The listing builds one solid part. Answer for the finished solid, in the listing's coordinates (mm). Face numbers are marked on the shaded views. Give positions to 0.01 mm unless a question says otherwise; leave off trailing zeros. Order: outer loops, then holes, each group sorted by start corner. A loop starts at its lowest first (then second) coordinate and runs counter-clockwise, first axis right, second up.
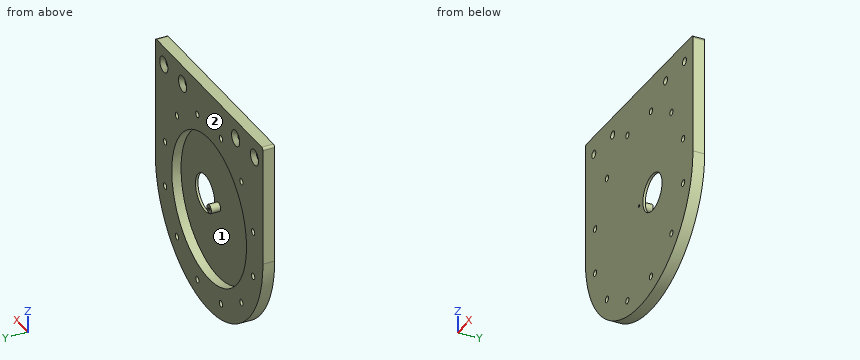
```python
from build123d import *

# Parameters (mm, degrees)
SKETCH1_R                                       = 1.27
BOSS_EXTRUDE1_DEPTH                             = 12.7
SKETCH2_R                                       = 79.375
SKETCH2_R_2                                     = 4.7625
CUT_EXTRUDE1_DEPTH                              = 10.033
SKETCH4_R                                       = 0.127
CUT_EXTRUDE2_DEPTH                              = 175.348445656
M8X1_25_TAPPED_HOLE1_D                          = 6.8
FILLET1_R                                       = 2.54
CSK_FOR_M8_FLAT_HEAD_MACHINE_SCREW3_D           = 8.4
CSK_FOR_M8_FLAT_HEAD_MACHINE_SCREW3_CSINK_D     = 17.3
CSK_FOR_M8_FLAT_HEAD_MACHINE_SCREW3_CSINK_ANGLE = 90
SKETCH22_R                                      = 20.346771346
CUT_EXTRUDE3_DEPTH                              = 175.174486052
F_6_32_TAPPED_HOLE2_D                           = 2.7051


with BuildPart() as part:
    # Sketch1 → Boss-Extrude1 (new body)
    with BuildSketch(Plane(origin=(0, 0, 0), x_dir=(1, 0, 0), z_dir=(0, 1, 0))):
        with BuildLine():
            Line((-114.3, 0), (-114.3, -131.040453687))
            Line((-114.3, -131.040453687), (114.3, -131.040453687))
            Line((114.3, -131.040453687), (114.3, 0))
            ThreePointArc((114.3, 0), (0, 114.3), (-114.3, 0))
        make_face()
        with Locations(Location((-68.474452923, 68.474452923, 0), (0, 0, 270))):
            Circle(SKETCH1_R, mode=Mode.SUBTRACT)
        with Locations(Location((25.06338928, 93.537842203, 0), (0, 0, 270))):
            Circle(SKETCH1_R, mode=Mode.SUBTRACT)
        with Locations(Location((68.474452923, 68.474452923, 0), (0, 0, 270))):
            Circle(SKETCH1_R, mode=Mode.SUBTRACT)
        with Locations(Location((93.537842203, 25.06338928, 0), (0, 0, 270))):
            Circle(SKETCH1_R, mode=Mode.SUBTRACT)
        with Locations(Location((93.537842203, -25.06338928, 0), (0, 0, 270))):
            Circle(SKETCH1_R, mode=Mode.SUBTRACT)
        with Locations(Location((68.474452923, -68.474452923, 0), (0, 0, 270))):
            Circle(SKETCH1_R, mode=Mode.SUBTRACT)
        with Locations(Location((25.06338928, -93.537842203, 0), (0, 0, 270))):
            Circle(SKETCH1_R, mode=Mode.SUBTRACT)
        with Locations(Location((-25.06338928, -93.537842203, 0), (0, 0, 270))):
            Circle(SKETCH1_R, mode=Mode.SUBTRACT)
        with Locations(Location((-68.474452923, -68.474452923, 0), (0, 0, 270))):
            Circle(SKETCH1_R, mode=Mode.SUBTRACT)
        with Locations(Location((-93.537842203, -25.06338928, 0), (0, 0, 270))):
            Circle(SKETCH1_R, mode=Mode.SUBTRACT)
        with Locations(Location((-93.537842203, 25.06338928, 0), (0, 0, 270))):
            Circle(SKETCH1_R, mode=Mode.SUBTRACT)
        with Locations(Location((-25.06338928, 93.537842203, 0), (0, 0, 270))):
            Circle(SKETCH1_R, mode=Mode.SUBTRACT)
        with Locations(Location((96.3, -111.040453687, 0), (0, 0, 270))):
            Circle(SKETCH1_R, mode=Mode.SUBTRACT)
        with Locations(Location((56.3, -111.040453687, 0), (0, 0, 270))):
            Circle(SKETCH1_R, mode=Mode.SUBTRACT)
        with Locations(Location((-56.3, -111.040453687, 0), (0, 0, 270))):
            Circle(SKETCH1_R, mode=Mode.SUBTRACT)
        with Locations(Location((-96.3, -111.040453687, 0), (0, 0, 270))):
            Circle(SKETCH1_R, mode=Mode.SUBTRACT)
    extrude(amount=BOSS_EXTRUDE1_DEPTH)

    # Sketch2 → Cut-Extrude1 (cut)
    with BuildSketch(Plane(origin=(0, 12.7, 0), x_dir=(1, 0, 0), z_dir=(0, 1, 0))):
        with Locations(Location((0, 0, 0), (0, 0, 270))):
            Circle(SKETCH2_R)
        with Locations(Location((0, 0, 0), (0, 0, 270))):
            Circle(SKETCH2_R_2, mode=Mode.SUBTRACT)
    extrude(amount=-CUT_EXTRUDE1_DEPTH, mode=Mode.SUBTRACT)

    # Sketch4 → Cut-Extrude2 (cut, through all)
    with BuildSketch(Plane(origin=(0, 12.7, 0), x_dir=(1, 0, 0), z_dir=(0, 1, 0))):
        with Locations(Location((0, 0, 0), (0, 0, 270))):
            Circle(SKETCH4_R)
    extrude(amount=-CUT_EXTRUDE2_DEPTH, mode=Mode.SUBTRACT)

    # M8x1.25 Tapped Hole1 (through all)
    with Locations(Plane(origin=(0, 12.7, 0), x_dir=(1, 0, 0), z_dir=(0, 1, 0))):
        with Locations((-93.537842203, 25.06338928), (-93.537842203, -25.06338928), (-25.06338928, 93.537842203), (-68.474452923, 68.474452923), (25.06338928, 93.537842203), (68.474452923, 68.474452923), (93.537842203, 25.06338928), (93.537842203, -25.06338928), (68.474452923, -68.474452923), (25.06338928, -93.537842203), (-25.06338928, -93.537842203), (-68.474452923, -68.474452923)):
            Hole(M8X1_25_TAPPED_HOLE1_D / 2)

    # Fillet1
    fillet1_edges = [part.edges().sort_by_distance(p)[0] for p in [
        (114.3, 6.35, 131.040453687),
        (-114.3, 6.35, 131.040453687),
    ]]
    fillet(fillet1_edges, radius=FILLET1_R)

    # CSK for M8 Flat Head Machine Screw3 (through all)
    with Locations(Plane(origin=(0, 12.7, 0), x_dir=(1, 0, 0), z_dir=(0, 1, 0))):
        with Locations((-96.3, -111.040453687), (-56.3, -111.040453687), (56.3, -111.040453687), (96.3, -111.040453687)):
            CounterSinkHole(CSK_FOR_M8_FLAT_HEAD_MACHINE_SCREW3_D / 2, CSK_FOR_M8_FLAT_HEAD_MACHINE_SCREW3_CSINK_D / 2, counter_sink_angle=CSK_FOR_M8_FLAT_HEAD_MACHINE_SCREW3_CSINK_ANGLE)

    # Sketch22 → Cut-Extrude3 (cut, through all)
    with BuildSketch(Plane(origin=(0, 2.667, 0), x_dir=(1, 0, 0), z_dir=(0, 1, 0))):
        with Locations(Location((28.284271346, 0, 0), (0, 0, 270))):
            Circle(SKETCH22_R)
    extrude(amount=-CUT_EXTRUDE3_DEPTH, mode=Mode.SUBTRACT)

    # #6-32 Tapped Hole2 (through all)
    with Locations(Plane(origin=(0, 12.7, 0), x_dir=(1, 0, 0), z_dir=(0, 1, 0))):
        with Locations((0, 0)):
            Hole(F_6_32_TAPPED_HOLE2_D / 2)


solid = part.part
```
1) Find section C-C (x = -69). Write down the section's boundary in (y, z).
Geometry says:
outline: (0, -91.12) - (12.7, -91.12) - (12.7, -71.83) - (0, -71.83) - close; (0, -65.12) - (12.7, -65.12) - (12.7, -39.24) - (2.67, -39.24) - (2.67, 39.24) - (12.7, 39.24) - (12.7, 65.12) - (0, 65.12) - close; (0, 71.83) - (12.7, 71.83) - (12.7, 131.04) - (0, 131.04) - close
2) Find section B-B (x = 56.3). Write down the section's boundary in (y, z), then the cut area to 3 significant figures.
Geometry says:
outline: (0, -99.47) - (12.7, -99.47) - (12.7, -55.95) - (2.67, -55.95) - (2.67, 55.95) - (12.7, 55.95) - (12.7, 102.39) - (8.25, 106.84) - (0, 106.84) - close; (0, 115.24) - (8.25, 115.24) - (12.7, 119.69) - (12.7, 131.04) - (0, 131.04) - close
area: 1,680 mm2
3) Straight lines are drawn through the part: probe 1 along X at (y, z) = (11.75, 93); probe 2 along Z at (x, y) = (56.3, 2.75); probe 3 along X at (y, z) = (12, 113). For each, find the intervals that lie inside material, in ascending order.
Geometry says:
probe 1: x = -114.3 to -28.42, -21.71 to 21.71, 28.42 to 114.3
probe 2: z = -99.47 to -55.95, 55.95 to 106.84, 115.24 to 131.04
probe 3: x = -114.3 to -104, -88.6 to -64, -48.6 to 48.6, 64 to 88.6, 104 to 114.3
4) For a pull along Z with two mould halves and no side action, classify the marked faces 1 and 2 as +Z half, -Z half, draft (parallel to the pull), parting line (faces both ways), or undercut.
Geometry says:
face 1: undercut
face 2: draft
5) Find section D-D (x = -42.5). Write down the section's boundary in (y, z), then the cut area to 3 significant figures.
Geometry says:
outline: (0, -106.1) - (12.7, -106.1) - (12.7, -67.04) - (2.67, -67.04) - (2.67, 67.04) - (12.7, 67.04) - (12.7, 131.04) - (0, 131.04) - close
area: 1,670 mm2
6) Given P1, Ø9, axis at x = 68.47, z = 68.47, coming from the -Y side; P2, Ø1, axis at x = 54, y = 11, coming from the -Z side; P3, Ø5, axis at y = 8, z = -84.5, coming from the +X side; P4, Ø5, axis at x = -50.5, y = 9.5, coming from the -Z side, each flat-ended and moving along its own axis, determine where each tip first touches the part or whether it passes through.
Geometry says:
P1: stops at y = 0
P2: stops at z = -101.01
P3: stops at x = 79.63
P4: stops at z = -103.73
7) Find section A-A (y = 6). Count the separate pieces of the cut face and the enclosed holes in it, then the cut area to 3 significant figures.
Geometry says:
separate pieces: 2
enclosed holes: 18
area: 30,100 mm2
